Geometry check sheet. Reference: the model listing, model coordinates, mm. A direction names the side the tool comes from. Give positions to 0.01 mm unless a question says otherwise; leave off trailing zeros. Write each loop counter-clockwise with the first axis right and the second up, starting at its lowest first coordinate (ties: lowest second). Pieces come first, ordered by that corner, then holes. Notation, with made-up numbers: M 11,-11.5 L 57,-11.5 A7 ccw 57,-7.5 Z; hole C -21,-40 d8. An arc over 180 degrees is marked long. One line per item, written item: value. Start each with the question number.
1. Cross-section at C-C on z = 3. Record the cut outline in (x, y).
2. Tool access check on faces 1 (the face through (8, 9, 4)), 2 (the face through (-1.9, 0.08, 4.28)). Record the directions out of +Z, -Z, +X, -X, +Y, -Y that give a thin tool (end or side, any length) a straight path to the whole face; none if there is none.
3. Release check for a two-part mould opening along X. For faces 3 (the face through (3.233, -1.341, 6.754)), 4 (the face through (-9, 8, 4)), 5 (the face through (0, 0, 0)) record: pulls with the +X half, pulls with the -X half, needs draft (parallel to the pull), parting line crosses it, or undercut.
4. Scan lines: line 1 (Y direction, x = 0, z = 5.35); line 2 (Y direction, x = -5.25, z = 5.5); line 3 (Y direction, x = 0, z = 6.8). Record each from-to range of solid material in increasing order.
5. Cross-section at D-D on z = 1.75. Record the cut outline in (x, y), then the cut area to 3 significant figures.
6. Gauge pin test, flat ends, axial feed: pin 1 (2.5 mm diameter, centred on x = 0, y = 0, fed in from +Z); pin 2 (2 mm diameter, centred on x = 6.5, z = 4.5, fed in from +Y). Record the tip position at first contact, or that the pin passes through.
7. Cross-section at A-A on x = 0. Record the cut outline in (y, z).
from build123d import *

# Parameters (mm, degrees)
F0_W     = 20
F0_H     = 20
F1_DEPTH = 7
F2_R     = 1.9
F3_DEPTH = 5
F4_R     = 3.5
F5_DEPTH = 0.5
F6_R     = 5


with BuildPart() as f1:
    # F0 (on Top) → F1 (new body)
    with BuildSketch(Plane.XY):
        Rectangle(F0_W, F0_H)
    extrude(amount=F1_DEPTH)

    # F2 (on face) → F3 (cut)
    with BuildSketch(Plane.XY.offset(7)):
        Circle(F2_R)
    extrude(amount=-F3_DEPTH, mode=Mode.SUBTRACT)

    # F4 (on face) → F5 (cut)
    with BuildSketch(Plane.XY.offset(7)):
        Circle(F4_R)
    extrude(amount=-F5_DEPTH, mode=Mode.SUBTRACT)

    # F6
    f6_edges = [f1.edges().sort_by_distance(p)[0] for p in [
        (-10, -10, 3.5),
        (10, -10, 3.5),
        (10, 10, 3.5),
        (-10, 10, 3.5),
    ]]
    fillet(f6_edges, radius=F6_R)


solid = f1.part
Report:
1. outline: M -10,-5 A5 ccw -5,-10 L 5,-10 A5 ccw 10,-5 L 10,5 A5 ccw 5,10 L -5,10 A5 ccw -10,5 Z; hole C 0,0 d3.8
2. face 1: +Z, -Z, +X, +Y
2. face 2: +Z
3. face 3: undercut
3. face 4: pulls with the -X half
3. face 5: needs draft
4. line 1: y = -10 to -1.9, 1.9 to 10
4. line 2: y = -9.99 to 9.99
4. line 3: y = -10 to -3.5, 3.5 to 10
5. outline: M -10,-5 A5 ccw -5,-10 L 5,-10 A5 ccw 10,-5 L 10,5 A5 ccw 5,10 L -5,10 A5 ccw -10,5 Z
5. area: 379 mm^2
6. pin 1: stops at z = 2
6. pin 2: stops at y = 9.97
7. outline: M -10,0 L 10,0 L 10,7 L 3.5,7 L 3.5,6.5 L 1.9,6.5 L 1.9,2 L -1.9,2 L -1.9,6.5 L -3.5,6.5 L -3.5,7 L -10,7 Z
